The model under review builds one solid part; all positions refer to its coordinate system, in mm. A direction names the side the tool comes from. Round coordinates to 2 decimals unless told otherwise and drop trailing zeros. Loops run counter-clockwise (first coordinate to the right, second up) from the corner with the lowest first, then second, coordinate; pieces in that order, holes last. Notation, with made-up numbers: M -38,-37.75 L 18,-37.75 A8 ccw 18,-27.75 Z; hole C -36,-28.75 d3. An arc over 180 degrees is marked long. Answer as a JSON object with one key per item and string values. Group by question number.
Item 1: Consider section D-D (z = 0). Give the boundary of the cut face in (x, y), and give its area (3 significant figures).
Item 2: Consider section C-C (y = -2). Give the boundary of the cut face in (x, z).
Item 3: Consider section A-A (x = 13). Give the boundary of the cut face in (y, z).
Item 4: Tool access review of faces 4 (the face through (10.56, -1.48, -0.54)), 5 (the face through (2.65, 3.06, 0)): name each direction out of +Z, -Z, +X, -X, +Y, -Y from which nothing blocks a thin tool from reaching the whole face with its end or side.
Item 5: The part is to be moulded in two halves that separate along X. For faces 1 (the face through (0, 7, 3)), 2 (the face through (-2.65, 3.06, 0.03)), 3 (the face through (1.802, 4.465, 5.723)), say which applies: +X half, -X half, draft (parallel to the pull), parting line (faces both ways), or undercut.
Item 6: Consider section B-B (y = 3.5). Give the boundary of the cut face in (x, z), and give its area (3 significant figures).
Item 7: Insertion check: P1, Ø1.5, axis at x = -14, z = 6.5, coming from the +Y side; P2, Ø5, axis at x = 9, y = 1, coming from the -Z side; P3, Ø1.7, axis at x = 0.5, z = 0, coming from the +Y side. Each pin has a flat end and moves straight along its axis. Give the tip position at first contact, or say it passes through.
Item 8: To check wall thickness, follow line 1 (X direction, y = -2.05, z = 0); line 2 (Y direction, x = 0, z = -15); line 3 (Z direction, x = -0.5, y = 6.75). State the ranges of each line that lie inside material, in increasing order.
```python
from build123d import *

# Parameters (mm, degrees)
SKETCH1_R           = 6
BOSS_EXTRUDE6_DEPTH = 7
SKETCH5_R           = 18
BOSS_EXTRUDE7_DEPTH = 3
CUT_EXTRUDE2_DEPTH  = 6
FILLET1_R           = 2
SKETCH8_R           = 2.5
CUT_EXTRUDE3_DEPTH  = 6
CUT_EXTRUDE4_DEPTH  = 8


with BuildPart() as part:
    # Sketch1 → Boss-Extrude6 (new body)
    with BuildSketch(Plane(origin=(0, 0, 0), x_dir=(1, 0, 0), z_dir=(0, 1, 0))):
        with Locations(Location((0, 0, 0), (0, 0, 270))):
            Circle(SKETCH1_R)
    extrude(amount=BOSS_EXTRUDE6_DEPTH)

    # Sketch5 → Boss-Extrude7 (add)
    with BuildSketch(Plane(origin=(0, 0, 0), x_dir=(-1, 0, 0), z_dir=(0, -1, 0))):
        with Locations(Location((0, 0, 0), (0, 0, 90))):
            Circle(SKETCH5_R)
    extrude(amount=BOSS_EXTRUDE7_DEPTH)

    # Sketch6 → Cut-Extrude2 (cut)
    with BuildSketch(Plane(origin=(0, 7, 0), x_dir=(1, 0, 0), z_dir=(0, 1, 0))):
        with BuildLine():
            Line((1.932582761, 1.5), (-1.932582761, 1.5))
            ThreePointArc((-1.932582761, 1.5), (-1.93394777, 1.498239684), (-1.935311176, 1.496478126))
            ThreePointArc((-1.935311176, 1.496478126), (-2.446399634, -0.002227546), (-1.932582761, -1.5))
            Line((-1.932582761, -1.5), (1.932582761, -1.5))
            ThreePointArc((1.932582761, -1.5), (2.446400648, 0), (1.932582761, 1.5))
        make_face()
    extrude(amount=-CUT_EXTRUDE2_DEPTH, mode=Mode.SUBTRACT)

    # Fillet1
    fillet1_edges = [part.edges().sort_by_distance(p)[0] for p in [
        (0, 0, -6),
    ]]
    fillet(fillet1_edges, radius=FILLET1_R)

    # Sketch8 → Cut-Extrude3 (cut)
    with BuildSketch(Plane(origin=(0, 0, 0), x_dir=(1, 0, 0), z_dir=(0, 1, 0))):
        with Locations(Location((13, 0, 0), (0, 0, 270))):
            Circle(SKETCH8_R)
        with Locations(Location((-13, 0.022078195, 0), (0, 0, 270))):
            Circle(SKETCH8_R)
    extrude(amount=-CUT_EXTRUDE3_DEPTH, mode=Mode.SUBTRACT)

    # Sketch9 → Cut-Extrude4 (cut)
    with BuildSketch(Plane(origin=(0, 7, 0), x_dir=(1, 0, 0), z_dir=(0, 1, 0))):
        with BuildLine():
            Line((-2.004154278, 1.733743242), (2.043845612, 1.686770617))
            ThreePointArc((2.043845612, 1.686770617), (2.649821606, -0.03074829), (2.004154278, -1.733743242))
            Line((2.004154278, -1.733743242), (-2.004154278, -1.733743242))
            ThreePointArc((-2.004154278, -1.733743242), (-2.65, 0), (-2.004154278, 1.733743242))
        make_face()
    extrude(amount=-CUT_EXTRUDE4_DEPTH, mode=Mode.SUBTRACT)


solid = part.part
```
Geometry results:
{
 "1": {"outline": "M -18,-3 L -15.5,-3 L -15.5,0 L -18,0 Z; M -10.5,-3 L 10.5,-3 L 10.5,0 L 8,0 A2 cw 6,2 L 6,7 L 2.65,7 L 2.65,-1 L -2.65,-1 L -2.65,7 L -6,7 L -6,2 A2 cw -8,0 L -10.5,0 Z; M 15.5,-3 L 18,-3 L 18,0 L 15.5,0 Z", "area": "121 mm^2"},
 "2": {"outline": "C 0,0 d36; hole C -13,-0.02 d5; hole C 13,0 d5"},
 "3": {"outline": "M -3,-12.45 L 0,-12.45 L 0,-2.5 L -3,-2.5 Z; M -3,2.5 L 0,2.5 L 0,12.45 L -3,12.45 Z"},
 "4": {"face 4": "+Y, -Y", "face 5": "+Y"},
 "5": {"face 1": "draft", "face 2": "undercut", "face 3": "parting line"},
 "6": {"outline": "C 0,0 d12; hole M -2,-1.73 L 2.04,-1.69 A2.65 ccw 2,1.73 L -2,1.73 A2.65 ccw Z", "area": "96.2 mm^2"},
 "7": {"P1": "stops at y = 0", "P2": "stops at z = -16.7", "P3": "stops at y = -1"},
 "8": {"line 1": "x = -18 to -15.5, -10.5 to 10.5, 15.5 to 18", "line 2": "y = -3 to 0", "line 3": "z = -5.98 to -1.72, 1.73 to 5.98"}
}
